Geometry check sheet. Reference: the model listing, model coordinates, mm. A direction names the side the tool comes from. Round coordinates to 2 decimals unless told otherwise and drop trailing zeros. Order: outer loops, then holes, each group sorted by start corner. A loop starts at its lowest first (then second) coordinate and runs counter-clockwise, first axis right, second up. Notation, with made-up numbers: (49.5, 76) -> (80.5, 76) arc R3 ccw to (80.5, 80) -> close; hole circle Ø3 at (72.25, 79). An arc over 180 degrees is marked (long way). Use a Markdown table: item, result. Add a question column.
Item 1: Gauge pin test, flat ends, axial feed: pin 1 Ø2 at (x, z) = (7.5, 51.5) entering from +Y; pin 2 Ø3 at (x, y) = (4.5, -19) entering from +Z; pin 3 Ø8 at (x, z) = (1.5, 21) entering from -Y. Record the tip position at first contact, or that the pin passes through.
Item 2: Mould release check, pull along X, two halves, no side actions. Record for faces 1 (the flat face through (-28.512, 0, 44)), 2 (the cylindrical face through (0.399, -0.61, 27.743)), 3 (the flat face through (-9.208, 26.7, 16.6)): pulls with the +X half, pulls with the -X half, needs draft (parallel to the pull), parting line crosses it, or undercut.
Item 3: Material ranges on probe 1 along Y at (x, z) = (-14, 42.5); probe 2 along X at (y, z) = (-6, 64); probe 3 along Z at (x, y) = (23, 0.5) (3 decimals), recorded low to high. Write a range as [from, to].
Item 4: Sectioned sample at C-C, the plane z = 40.5. Record the cut outline in (x, y).
Item 5: Sectioned sample at D-D, the plane x = 3. Record the cut outline in (y, z), and give its area (3 significant figures).
Item 6: Set-up check for faces 4 (the flat face through (-26, 0, 71.564)), 5 (the flat face through (-22.162, 26.7, 16.6)), 6 (the cylindrical face through (-26.58, 12.116, 46.306)): record each of +Z, -Z, +X, -X, +Y, -Y from which the full face is reachable in a straight line by a thin tool's end or side.
Item 7: Sectioned sample at B-B, the plane z = 60. Record the cut outline in (x, y).
from build123d import *
from build123d.topology import SkipClean

# Parameters (mm, degrees)
BOSS_EXTRUDE1_DEPTH                  = 28.5115
SKETCH5_W                            = 57.023
SKETCH5_H                            = 56.896
SKETCH5_W_2                          = 49.403
SKETCH5_H_2                          = 49.276
BOSS_EXTRUDE2_DEPTH                  = 40.64
BOSS_EXTRUDE2_DIRECTION_2_REACH      = 54.207
BOSS_EXTRUDE2_DIRECTION_2_END_RADIUS = 30.9245
CUT_EXTRUDE1_START                   = -12.954
CUT_EXTRUDE1_DEPTH                   = 12.954
CUT_EXTRUDE2_START                   = -12.954
CUT_EXTRUDE2_DEPTH                   = 12.954
CUT_EXTRUDE3_DEPTH                   = 3.81
BOSS_EXTRUDE3_REACH                  = 59.717
BOSS_EXTRUDE3_END_RADIUS             = 30.9245
SKETCH11_W                           = 15.875
SKETCH11_H                           = 53.086
BOSS_EXTRUDE5_DEPTH                  = 16.764
BOSS_EXTRUDE6_DEPTH                  = 16.764
CUT_EXTRUDE4_START                   = -3.81
CUT_EXTRUDE4_OUTLINE_R               = 2.159
CUT_EXTRUDE4_DEPTH                   = 3.81


# Read off the part's stored shape, not the designer's step: Cut-Extrude4
with BuildPart() as part:
    # Sketch2 → Boss-Extrude1 (new, symmetric)
    with BuildSketch(Plane(origin=(0, 0, 0), x_dir=(0, 0, -1), z_dir=(1, 0, 0))):
        with BuildLine():
            Line((0, -30.9245), (0, -27.7495))
            ThreePointArc((0, -27.7495), (-27.7495, 0), (0, 27.7495))
            Line((0, 27.7495), (0, 30.9245))
            ThreePointArc((0, 30.9245), (-30.9245, 0), (0, -30.9245))
        make_face()
    extrude(amount=BOSS_EXTRUDE1_DEPTH, both=True)

    # Sketch5 → Boss-Extrude2 (add)
    with BuildSketch(Plane.XY.offset(30.9245)):
        Rectangle(SKETCH5_W, SKETCH5_H)
        Rectangle(SKETCH5_W_2, SKETCH5_H_2, mode=Mode.SUBTRACT)
    extrude(amount=BOSS_EXTRUDE2_DEPTH)

    # Boss-Extrude2 direction 2: up to this cylinder (the profile starts outside it)
    boss_extrude2_direction_2_end = Plane(origin=(0, 0, 0), z_dir=(-1, 0, 0)) * Cylinder(BOSS_EXTRUDE2_DIRECTION_2_END_RADIUS, 171.263, mode=Mode.PRIVATE)
    # Sketch5 → Boss-Extrude2 direction 2 (add, up to the surface)
    with BuildSketch(Plane.XY.offset(30.9245), mode=Mode.PRIVATE) as boss_extrude2_direction_2_sk1:
        Rectangle(SKETCH5_W, SKETCH5_H)
        Rectangle(SKETCH5_W_2, SKETCH5_H_2, mode=Mode.SUBTRACT)
    boss_extrude2_direction_2_tool1 = extrude(boss_extrude2_direction_2_sk1.sketch, amount=-BOSS_EXTRUDE2_DIRECTION_2_REACH, mode=Mode.PRIVATE) - boss_extrude2_direction_2_end
    add(boss_extrude2_direction_2_tool1.solids().sort_by_distance((0, 27.642471, 30.9245))[0])
    add(boss_extrude2_direction_2_tool1.solids().sort_by_distance((0, 27.642471, 30.9245))[1])

    # Sketch7 → Cut-Extrude1 (cut)
    with SkipClean():  # the faces are left unmerged after this step: merging them gives an invalid solid
        with BuildSketch(Plane.ZY.offset(-9.2075).offset(CUT_EXTRUDE1_START)):
            with BuildLine():
                Line((0, 30.9245), (0, 32.0421))
                ThreePointArc((0, 32.0421), (32.0421, 0), (0, -32.0421))
                Line((0, -32.0421), (0, -30.9245))
                ThreePointArc((0, -30.9245), (30.9245, 0), (0, 30.9245))
            make_face()
        extrude(amount=CUT_EXTRUDE1_DEPTH, mode=Mode.SUBTRACT)

    # Sketch8 → Cut-Extrude2 (cut)
    with SkipClean():  # the faces are left unmerged after this step: merging them gives an invalid solid
        with BuildSketch(Plane(origin=(-9.2075, 0, 0), x_dir=(0, 0, -1), z_dir=(1, 0, 0)).offset(CUT_EXTRUDE2_START)):
            with BuildLine():
                Line((0, 30.9245), (0, 32.0421))
                ThreePointArc((0, 32.0421), (-32.0421, 0), (0, -32.0421))
                Line((0, -32.0421), (0, -30.9245))
                ThreePointArc((0, -30.9245), (-30.9245, 0), (0, 30.9245))
            make_face()
        extrude(amount=CUT_EXTRUDE2_DEPTH, mode=Mode.SUBTRACT)

    # Sketch10 → Cut-Extrude3 (cut)
    with SkipClean():  # the faces are left unmerged after this step: merging them gives an invalid solid
        with BuildSketch(Plane(origin=(28.5115, 0, 0), x_dir=(0, 0, -1), z_dir=(1, 0, 0))):
            with BuildLine():
                Line((-56.8071, 24.638), (-71.5645, 24.638))
                Line((-71.5645, 24.638), (-71.5645, 8.128))
                Line((-71.5645, 8.128), (-56.8071, 8.128))
                ThreePointArc((-56.8071, 8.128), (-48.5521, 16.383), (-56.8071, 24.638))
            make_face()
        extrude(amount=-CUT_EXTRUDE3_DEPTH, mode=Mode.SUBTRACT)

    # Boss-Extrude3: up to this cylinder (the profile starts outside it)
    with SkipClean():  # the faces are left unmerged after this step: merging them gives an invalid solid
        boss_extrude3_end = Plane(origin=(0, 0, 0), z_dir=(-1, 0, 0)) * Cylinder(BOSS_EXTRUDE3_END_RADIUS, 182.283, mode=Mode.PRIVATE)
        # Sketch11 → Boss-Extrude3 (add, up to the surface)
        with BuildSketch(Plane.XY.offset(32.0421), mode=Mode.PRIVATE) as boss_extrude3_sk1:
            with Locations((0, -1.905)):
                Rectangle(SKETCH11_W, SKETCH11_H)
        boss_extrude3_tool1 = extrude(boss_extrude3_sk1.sketch, amount=-BOSS_EXTRUDE3_REACH, mode=Mode.PRIVATE) - boss_extrude3_end
        add(boss_extrude3_tool1.solids().sort_by_distance((0, -1.905, 32.0421))[0])

    # Sketch15 → Boss-Extrude5 (add)
    with SkipClean():  # the faces are left unmerged after this step: merging them gives an invalid solid
        with BuildSketch(Plane.ZY.offset(7.9375)):
            Polygon((32.0421, -24.638), (24.653467357, -24.638), (32.0421, -10.668), align=None)
            Polygon((24.653467357, 24.638), (32.0421, 10.668), (32.0421, 24.638), align=None)
        extrude(amount=BOSS_EXTRUDE5_DEPTH)

    # Sketch16 → Boss-Extrude6 (add)
    with SkipClean():  # the faces are left unmerged after this step: merging them gives an invalid solid
        with BuildSketch(Plane(origin=(7.9375, 0, 0), x_dir=(0, 0, -1), z_dir=(1, 0, 0))):
            Polygon((-32.0421, -24.638), (-24.653467357, -24.638), (-32.0421, -10.668), align=None)
            Polygon((-24.653467357, 24.638), (-32.0421, 10.668), (-32.0421, 24.638), align=None)
        extrude(amount=BOSS_EXTRUDE6_DEPTH)

    # Cut-Extrude4 outline → Cut-Extrude4 (cut)
    with SkipClean():  # the faces are left unmerged after this step: merging them gives an invalid solid
        with BuildSketch(Plane.ZY.offset(28.5115).offset(CUT_EXTRUDE4_START)):
            with Locations((46.7741, -13.716)):
                Circle(CUT_EXTRUDE4_OUTLINE_R)
            with Locations((46.7741, 14.224)):
                Circle(CUT_EXTRUDE4_OUTLINE_R)
        extrude(amount=CUT_EXTRUDE4_DEPTH, mode=Mode.SUBTRACT)


solid = part.part
Found:
| question | item | result |
|---|---|---|
| 1 | pin 1 | stops at y = 28.45 |
| 1 | pin 2 | stops at z = 32.04 |
| 1 | pin 3 | stops at y = -28.45 |
| 2 | face 1 | pulls with the -X half |
| 2 | face 2 | needs draft |
| 2 | face 3 | undercut |
| 3 | probe 1 | y = [-28.45, -24.64], [24.64, 28.45] |
| 3 | probe 2 | x = [-28.51, -24.7], [24.7, 28.51] |
| 3 | probe 3 | z = [27.745, 30.92] |
| 4 | outline | (-28.51, -28.45) -> (28.51, -28.45) -> (28.51, 28.45) -> (-28.51, 28.45) -> close; hole (-24.7, -24.64) -> (24.7, -24.64) -> (24.7, 24.64) -> (-24.7, 24.64) -> close |
| 5 | outline | (-30.92, 0) -> (-27.75, 0) arc R27.75 cw to (27.75, 0) -> (30.92, 0) arc R30.92 ccw to (28.45, 12.13) -> (28.45, 71.56) -> (24.64, 71.56) -> (24.64, 32.04) -> (-24.64, 32.04) -> (-24.64, 71.56) -> (-28.45, 71.56) -> (-28.45, 12.13) arc R30.92 ccw to start |
| 5 | area | 955 mm2 |
| 6 | face 4 | +Z, +X, -X, +Y, -Y |
| 6 | face 5 | none |
| 6 | face 6 | -X |
| 7 | outline | (-28.51, -28.45) -> (28.51, -28.45) -> (28.51, 8.13) -> (24.7, 8.13) -> (24.7, -24.64) -> (-24.7, -24.64) -> (-24.7, 24.64) -> (28.51, 24.64) -> (28.51, 28.45) -> (-28.51, 28.45) -> close |
